Input: dimensioned drawing with shaded views. Units: mm. Origin: part minimum x, y, z. A direction names the side the tool comes from. Round coordinates to 2 decimals unless told otherwise and drop trailing zeros. Loops run counter-clockwise (first coordinate to the right, second up) from the corner with the lowest first, then second, coordinate; pieces in that order, holes last. Notation, with made-up numbers: M 22.5,-27 L 40.5,-27 A23 ccw 40.5,-7 Z; hole C 34,14 d5. An arc over 180 degrees is marked long. Write each question's results on one line, items separated by ' | '. Start each with the question number.
1. Section D-D on x = 36. Output: boundary loops of the cut face in (y, z).
2. Draft query along Y for the marked faces 4, 5 and 6. Return one class per face: released by +Y, released by -Y, zero draft, split by the parting line, or undercut.
3. Contact query for flat-ended pins moving along their axis: pin 1 Ø5 at (x, y) = (16, 58) entering from +Z; pin 2 Ø10 at (x, y) = (40, 57.5) entering from -Z; pin 3 Ø11 at (y, z) = (74, 40) entering from +X; pin 4 Ø2 at (x, y) = (25, 24.5) entering from -Z. Output: stop coordinate, or through.
4. Section A-A on y = 30.5. Output: boundary loops of the cut face in (x, z).
5. Section B-B on y = 6. Output: boundary loops of the cut face in (x, z).
6. Set-up query: the marked faces 1, 2 and 3. Return all of +Z, -Z, +X, -X, +Y, -Y with unobstructed straight access to the full face (end or side cutting, diameter ignored); none if empty.
7. Ray query, line 1 (Y direction, x = 5, z = 40); line 2 (Y direction, x = 25, z = 7); line 3 (Z direction, x = 15.5, y = 63.5). Return the intervals inside material, ascending.
8. Section C-C on z = 33.5. Output: boundary loops of the cut face in (x, y).
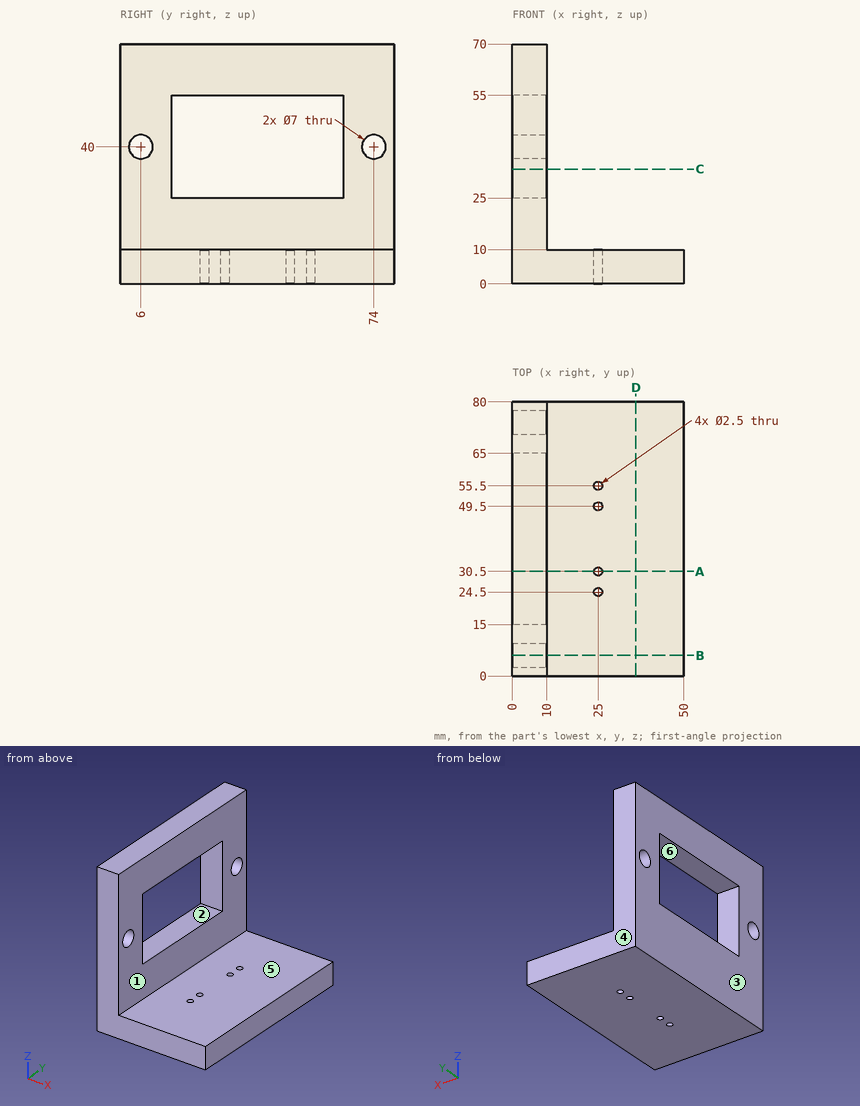
Taken from the geometry:
1) outline: M 0,0 L 80,0 L 80,10 L 0,10 Z
2) face 4: released by +Y | face 5: zero draft | face 6: undercut
3) pin 1: z = 10 | pin 2: z = 0 | pin 3: x = 10 | pin 4: through
4) outline: M 0,0 L 23.75,0 L 23.75,10 L 10,10 L 10,25 L 0,25 Z; M 0,55 L 10,55 L 10,70 L 0,70 Z; M 26.25,0 L 50,0 L 50,10 L 26.25,10 Z
5) outline: M 0,0 L 50,0 L 50,10 L 10,10 L 10,36.5 L 0,36.5 Z; M 0,43.5 L 10,43.5 L 10,70 L 0,70 Z
6) face 1: +Z, +X, +Y, -Y | face 2: +X, -X | face 3: +Z, -Z, -X, +Y, -Y
7) line 1: 0 to 2.5, 9.5 to 15, 65 to 70.5, 77.5 to 80 | line 2: 0 to 23.25, 25.75 to 29.25, 31.75 to 48.25, 50.75 to 54.25, 56.75 to 80 | line 3: 0 to 10
8) outline: M 0,0 L 10,0 L 10,15 L 0,15 Z; M 0,65 L 10,65 L 10,80 L 0,80 Z
